Design review of the part built by this model. Coordinates are the model's own, in mm. Face numbers are marked on the shaded views. A direction names the side the tool comes from. Give positions to 0.01 mm unless a question says otherwise; leave off trailing zeros. Order: outer loops, then holes, each group sorted by start corner. A loop starts at its lowest first (then second) coordinate and runs counter-clockwise, first axis right, second up. Notation, with made-up numbers: (80, 7) -> (113, 7) arc R8 ccw to (113, 15) -> close; hole circle Ø9 at (70, 77.25). An arc over 180 degrees is marked (long way). Use a Markdown table: item, result. Add a question column.
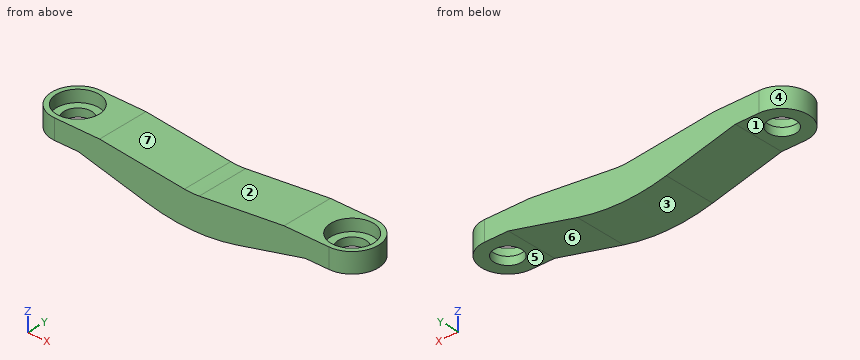
Solid Edge part; units mm, degrees
sketch "Sketch1" plane through (0, 0, 0) normal (0, 0, 1) x (1, 0, 0)
  line L0 (-48, 5.5) -> (10, 5.5)
  line L1 (-48, -5.5) -> (10, -5.5)
  arc A0 (-48, -5.5) -> (-48, 5.5) centre (-48, 0) cw
  arc A1 (10, 5.5) -> (10, -5.5) centre (10, 0) cw
extrude "Protrusion1" add sketch "Sketch1" along normal blind 20
sketch "Sketch2" plane through (0, 0, 20) normal (0, 0, 1) x (1, 0, 0)
  circle A0 centre (-48, 0) radius 4.5
extrude "Extrusionsausschnitt_1" cut sketch "Sketch2" against normal blind 2.5
sketch "Sketch3" plane through (0, 0, 20) normal (0, 0, 1) x (1, 0, 0)
  circle A0 centre (10, 0) radius 4.5
extrude "Extrusionsausschnitt_2" cut sketch "Sketch3" against normal blind 2.5
sketch "Sketch4" plane through (0, 0, 0) normal (0, -1, 0) x (1, 0, 0)
  line L0 (-38.5, 20) -> (-19, 17.9505)
  line L1 (0.5, 20) -> (-19, 17.9505)
extrude "Cutout1" cut sketch "Sketch4" along normal up to next and the other way up to next material side at (-28.7448, 0, 19.025)
sketch "Sketch5" plane through (0, 0, 0) normal (0, -1, 0) x (1, 0, 0)
  line L0 (59.3337, 10) -> (65.9133, -0.3822)
  line L1 (-60.6663, 10) -> (59.3337, 10)
  line L2 (-60.6663, 10) -> (-66.4669, -5.8923)
  dimension "D1" = 60.6663
extrude "Cutout2" cut sketch "Sketch5" along normal up to next and the other way up to next material side at (62.5813, 0, 4.7821)
hole "Bohrung_1" at (-48, 0, 10) direction (0, 0, 1) diameter 5.8 end up to next counterbore diameter 10 counterbore depth 5.8
hole "Hole1" at (10, 0, 10) direction (0, 0, 1) diameter 5.8 end up to next counterbore diameter 10 counterbore depth 5.8
sketch "Sketch6" plane through (0, 5.5, 15) normal (0, 1, 0) x (1, 0, 0)
  line L0 (5, -0.8) -> (-19, 5)
  line L1 (15.5, -0.8) -> (5, -0.8)
  line L2 (43.1446, 3.1504) -> (15.5, -0.8)
  line L3 (11.6347, 27.0505) -> (43.1446, 3.1504)
  line L4 (-73.2169, -0.8) -> (11.6347, 27.0505)
  line L5 (-43, -0.8) -> (-73.2169, -0.8)
  line L6 (-43, -0.8) -> (-19, 5)
  dimension "D1" = 5
  dimension "D2" = 43
  dimension "D3" = 5
extrude "Cutout3" cut sketch "Sketch6" against normal up to next
fillet "Verrundung_2" radius 40 1 edges at (-19, 0, 10)
fillet "Verrundung_3" radius 15 1 edges at (-19, 0, 17.9505)
properties part number "25" material "Polykarbonat"
1) Add section C-C (z = 19). Give the boundary of the cut face in (x, y), then the cut area to 3 significant figures.
2) Add section D-D (y = 3.75). Give the boundary of the cut face in (x, z), then the cut area to 3 significant figures.
3) For L1, parallel to X at y = 0, z = 17.15; L2, parallel to Y at x = -48, z = 19.3; L3, parallel to Y at x = 10, z = 16.85, list the stretches that pass through material, from the lowest coordinate up. Write a range as [from, to].
4) Machinability: for the marked faces 1, 2 and 3, which of the approach directions +Z, -Z, +X, -X, +Y, -Y give a long, thin tool a straight path to every point of the face, cutting with its end or side? Answer none if there is none.
5) Add section B-B (x = 9). Give the boundary of the cut face in (y, z), then the cut area to 3 significant figures.
6) Add section A-A (y = 0). Give the boundary of the cut face in (x, z), then the cut area to 3 significant figures.
7) The part is to be moulded in two halves that separate along X. For the marked faces 4, 5, 6 and 7, say which applies: +X half, -X half, draft (parallel to the pull), parting line (faces both ways), or undercut.
8) Insertion check: pin 1 (3 mm diameter, centred on x = -46.5, y = -1.5, fed in from -Z); pin 2 (1.5 mm diameter, centred on y = 1, z = 17, fed in from +X); pin 3 (1 mm diameter, centred on x = -35.5, y = 4.5, fed in from +Z). Each pin has a flat end and moves straight along its axis. Give the tip position at first contact, or say it passes through.
Worked answers:
| question | item | result |
|---|---|---|
| 1 | outline | (-48, -5.5) -> (-28.99, -5.5) -> (-28.99, 5.5) -> (-48, 5.5) arc R5.5 ccw to start; (-9.01, -5.5) -> (10, -5.5) arc R5.5 ccw to (10, 5.5) -> (-9.01, 5.5) -> close; hole circle Ø9 at (-48, 0); hole circle Ø9 at (10, 0) |
| 1 | area | 386 mm^2 |
| 2 | outline | (-52.02, 15.8) -> (-43, 15.8) -> (-28.4, 12.27) arc R40 ccw to (-9.6, 12.27) -> (5, 15.8) -> (14.02, 15.8) -> (14.02, 20) -> (12.49, 20) -> (12.49, 17.5) -> (7.51, 17.5) -> (7.51, 20) -> (0.5, 20) -> (-17.43, 18.12) arc R15 cw to (-20.57, 18.12) -> (-38.5, 20) -> (-45.51, 20) -> (-45.51, 17.5) -> (-50.49, 17.5) -> (-50.49, 20) -> (-52.02, 20) -> close |
| 2 | area | 345 mm^2 |
| 3 | L1 | [-53.5, -50.9], [-45.1, 7.1], [12.9, 15.5] |
| 3 | L2 | [-5.5, -4.5], [4.5, 5.5] |
| 3 | L3 | [-5.5, -2.9], [2.9, 5.5] |
| 4 | face 1 | -Z, -X, +Y, -Y |
| 4 | face 2 | +Z, +Y, -Y |
| 4 | face 3 | -Z, +Y, -Y |
| 5 | outline | (-5.5, 15.8) -> (-2.72, 15.8) -> (-2.72, 17.5) -> (-4.39, 17.5) -> (-4.39, 20) -> (-5.5, 20) -> close; (2.72, 15.8) -> (5.5, 15.8) -> (5.5, 20) -> (4.39, 20) -> (4.39, 17.5) -> (2.72, 17.5) -> close |
| 5 | area | 15.0 mm^2 |
| 6 | outline | (-53.5, 15.8) -> (-50.9, 15.8) -> (-50.9, 17.5) -> (-52.5, 17.5) -> (-52.5, 20) -> (-53.5, 20) -> close; (-45.1, 15.8) -> (-43, 15.8) -> (-28.4, 12.27) arc R40 ccw to (-9.6, 12.27) -> (5, 15.8) -> (7.1, 15.8) -> (7.1, 17.5) -> (5.5, 17.5) -> (5.5, 20) -> (0.5, 20) -> (-17.43, 18.12) arc R15 cw to (-20.57, 18.12) -> (-38.5, 20) -> (-43.5, 20) -> (-43.5, 17.5) -> (-45.1, 17.5) -> close; (12.9, 15.8) -> (15.5, 15.8) -> (15.5, 20) -> (14.5, 20) -> (14.5, 17.5) -> (12.9, 17.5) -> close |
| 6 | area | 317 mm^2 |
| 7 | face 4 | -X half |
| 7 | face 5 | draft |
| 7 | face 6 | +X half |
| 7 | face 7 | undercut |
| 8 | pin 1 | z = 15.8 |
| 8 | pin 2 | x = 15.49 |
| 8 | pin 3 | z = 19.74 |
